The model under review builds one solid part; all positions refer to its coordinate system, in mm. Face numbers are marked on the shaded views. A direction names the side the tool comes from. Give positions to 0.01 mm unless a question says otherwise; leave off trailing zeros. Order: outer loops, then holes, each group sorted by start corner. A loop starts at its lowest first (then second) coordinate and runs counter-clockwise, first axis right, second up. Notation, with made-up numbers: M 74,59 L 113,59 A12 ccw 113,75 Z; hole C 51,-15 d2. An arc over 180 degrees is marked long. One line per question, with ' | ' between items. Start each with the question number.
1. We need section D-D on z = -4. Write out the cut boundary in (x, y), then the cut area to 3 significant figures.
2. We need section B-B on z = -2.25. Write out the cut boundary in (x, y), then the cut area to 3 significant figures.
3. For the marked faces 1 and 2, list the 3-axis set-ups (+Z, -Z, +X, -X, +Y, -Y) from which the entire face can be reached by the end or side of a thin tool; tool diameter is ignored.
4. Wall thickness on L1, parallel to Z at x = 5.5, y = 0.25; L2, parallel to Z at x = 4.75, y = 0.15; L3, parallel to Z at x = 0, y = 0.15: over which ranges is each line inside the solid? List them lowest first.
5. We need section A-A on y = 0.15. Write out the cut boundary in (x, z).
6. The part is to be moulded in two halves that separate along X. For the marked faces 3, 4 and 5, say which applies: +X half, -X half, draft (parallel to the pull), parting line (faces both ways), or undercut.
7. We need section C-C on x = 0. Write out the cut boundary in (y, z), then the cut area to 3 significant figures.
8. Insertion check: P1, Ø0.5, axis at x = 5.5, y = 0, coming from the +Z side; P2, Ø1.9, axis at x = 5.55, z = -2, coming from the +Y side; P3, Ø0.5, axis at y = 0, z = -2.5, coming from the -X side. Each pin has a flat end and moves straight along its axis. Give the tip position at first contact, or say it passes through.
```python
from build123d import *

# Parameters (mm, degrees)
F0_R     = 0.6
F1_DEPTH = 0.5


with BuildPart() as f1:
    # F0 (on Front) → F1 (new body, symmetric)
    with BuildSketch(Plane.XZ):
        with BuildLine():
            Line((6.572272, 1), (6.99489, 1.906308))
            ThreePointArc((6.99489, 1.906308), (-7.25, 0), (6.99489, -1.906308))
            Line((6.99489, -1.906308), (6.572272, -1))
            Line((6.572272, -1), (5.072272, -1))
            Line((5.072272, -1), (4.649654, -1.906308))
            Line((4.649654, -1.906308), (4.649654, -2.906308))
            Line((4.649654, -2.906308), (5.076546, -3.645707))
            ThreePointArc((5.076546, -3.645707), (-6.25, 0), (5.076546, 3.645707))
            Line((5.076546, 3.645707), (4.649654, 2.906308))
            Line((4.649654, 2.906308), (4.649654, 1.906308))
            Line((4.649654, 1.906308), (5.072272, 1))
            Line((5.072272, 1), (6.572272, 1))
        make_face()
        with Locations((5.549654, -2)):
            Circle(F0_R, mode=Mode.SUBTRACT)
        with Locations((5.549654, 2)):
            Circle(F0_R, mode=Mode.SUBTRACT)
    extrude(amount=F1_DEPTH, both=True)


solid = f1.part
```
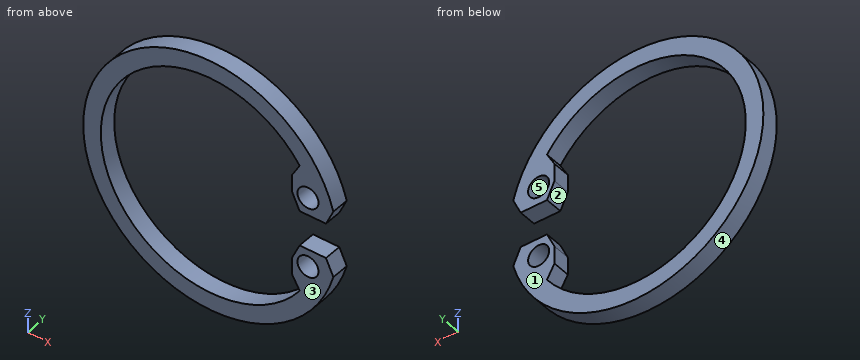
Entries:
1) outline: M -6.05,-0.5 L -4.8,-0.5 L -4.8,0.5 L -6.05,0.5 Z; M 4.8,-0.5 L 6.05,-0.5 L 6.05,0.5 L 4.8,0.5 Z | area: 2.49 mm^2
2) outline: M -6.89,-0.5 L -5.83,-0.5 L -5.83,0.5 L -6.89,0.5 Z; M 4.65,-0.5 L 5,-0.5 L 5,0.5 L 4.65,0.5 Z; M 6.1,-0.5 L 6.89,-0.5 L 6.89,0.5 L 6.1,0.5 Z | area: 2.21 mm^2
3) face 1: +Z, -Z, +X, -X, +Y | face 2: +Y, -Y
4) L1: z = -4.72 to -2.6, -1.4 to -1, 1 to 1.4, 2.6 to 4.72 | L2: z = -5.48 to -4.06, -3.08 to -1.69, 1.69 to 3.08, 4.06 to 5.48 | L3: z = -7.25 to -6.25, 6.25 to 7.25
5) outline: M 4.65,-2.91 L 5.08,-3.65 A6.25 cw long 5.08,3.65 L 4.65,2.91 L 4.65,1.91 L 5.07,1 L 6.57,1 L 6.99,1.91 A7.25 ccw long 6.99,-1.91 L 6.57,-1 L 5.07,-1 L 4.65,-1.91 Z; hole C 5.55,-2 d1.2; hole C 5.55,2 d1.2
6) face 3: draft | face 4: parting line | face 5: undercut
7) outline: M -0.5,-7.25 L 0.5,-7.25 L 0.5,-6.25 L -0.5,-6.25 Z; M -0.5,6.25 L 0.5,6.25 L 0.5,7.25 L -0.5,7.25 Z | area: 2.00 mm^2
8) P1: stops at z = 5 | P2: stops at y = 0.5 | P3: stops at x = -6.89
